Design review of the part built by this model. Coordinates are the model's own, in mm. Face numbers are marked on the shaded views. A direction names the side the tool comes from. Round coordinates to 2 decimals unless told otherwise and drop trailing zeros. Loops run counter-clockwise (first coordinate to the right, second up) from the corner with the lowest first, then second, coordinate; pieces in that order, holes last. Notation, with made-up numbers: (-5.75, -8.5) - (44.25, -8.5) arc R25 cw to (44.25, 26.5) - close; hole circle Ø11 at (35, 39.25). An arc over 180 degrees is marked (long way). Return JSON: item names as keys, results as strings. Group by question number.
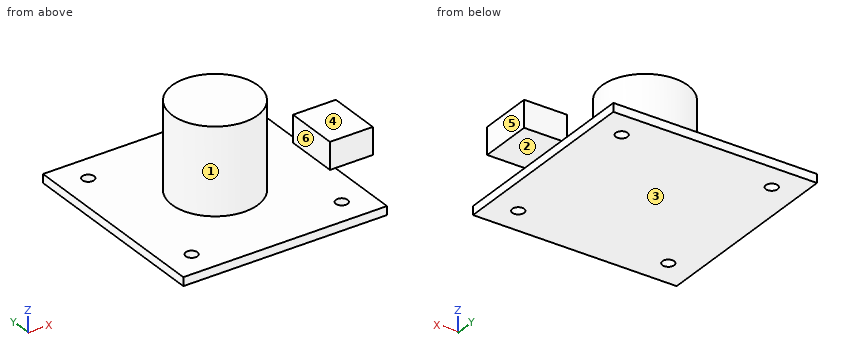
from build123d import *

# Parameters (mm, degrees)
SKETCH_1_W        = 38
SKETCH_1_H        = 38
SKETCH_1_R        = 1.1
USB_38_PCB_DEPTH  = 1.6
EXTRUDE_START     = 1.6
SKETCH_2_R        = 8
EXTRUDE_M12_DEPTH = 16
USB_START         = 1.6
SKETCH_3_W        = 8
SKETCH_3_H        = 10
USB_DEPTH         = 5


with BuildPart() as part:
    # 草图1 → USB摄像头38方PCB占位 (new body)
    with BuildSketch(Plane.XY):
        Rectangle(SKETCH_1_W, SKETCH_1_H)
        with Locations((-14, -14)):
            Circle(SKETCH_1_R, mode=Mode.SUBTRACT)
        with Locations((-14, 14)):
            Circle(SKETCH_1_R, mode=Mode.SUBTRACT)
        with Locations((14, -14)):
            Circle(SKETCH_1_R, mode=Mode.SUBTRACT)
        with Locations((14, 14)):
            Circle(SKETCH_1_R, mode=Mode.SUBTRACT)
    extrude(amount=USB_38_PCB_DEPTH)

    # 草图2 → M12镜头占位 (add)
    with BuildSketch(Plane.XY.offset(EXTRUDE_START)):
        Circle(SKETCH_2_R)
    extrude(amount=EXTRUDE_M12_DEPTH)

    # 草图3 → USB插头接口占位 (add)
    with BuildSketch(Plane.XY.offset(USB_START)):
        with Locations((22, 0)):
            Rectangle(SKETCH_3_W, SKETCH_3_H)
    extrude(amount=USB_DEPTH)


solid = part.part
Q1. Insertion check: pin 1 Ø0.5 at (y, z) = (2, 1) entering from +X; pin 2 Ø4 at (x, y) = (21.5, -1.5) entering from +Z; pin 3 Ø2.5 at (y, z) = (0, 5) entering from -X; pin 4 Ø7.5 at (x, y) = (21, 0) entering from -Z. Each pin has a flat end and moves straight along its axis. Give the tip position at first contact, or say it passes through.
Q2. Add section D-D, the plane y = 0. State the section outline as (x, z) points, plus the area to 3 significant figures.
Q3. Add section A-A, the plane y = 14. State the section outline as (x, z) points, plus the area to 3 significant figures.
Q4. Draft analysis for pull direction X (two halves, no side actions). For the marked faces 4, 5 and 6, state which applies: pulls with the +X half, pulls with the -X half, needs draft (parallel to the pull), parting line crosses it, or undercut.
Q5. Add section C-C, the plane z = 4.75. State the section outline as (x, y) points.
Q6. Tool access review of the marked faces 1, 2 and 3: name each direction out of +Z, -Z, +X, -X, +Y, -Y from which nothing blocks a thin tool from reaching the whole face with its end or side.
Q7. For line 1 (Y direction, x = -14, z = 0.95); line 2 (Z direction, x = 18, y = 13); line 3 (Z direction, x = 21, y = -2.5), list the stretches that pass through material, from the lowest coordinate up.
Evaluation:
{
 "1": {"pin 1": "x = 19", "pin 2": "z = 6.6", "pin 3": "x = -8", "pin 4": "z = 0"},
 "2": {"outline": "(-19, 0) - (19, 0) - (19, 1.6) - (26, 1.6) - (26, 6.6) - (18, 6.6) - (18, 1.6) - (8, 1.6) - (8, 17.6) - (-8, 17.6) - (-8, 1.6) - (-19, 1.6) - close", "area": "357 mm²"},
 "3": {"outline": "(-19, 0) - (-15.1, 0) - (-15.1, 1.6) - (-19, 1.6) - close; (-12.9, 0) - (12.9, 0) - (12.9, 1.6) - (-12.9, 1.6) - close; (15.1, 0) - (19, 0) - (19, 1.6) - (15.1, 1.6) - close", "area": "53.8 mm²"},
 "4": {"face 4": "needs draft", "face 5": "pulls with the +X half", "face 6": "undercut"},
 "5": {"outline": "circle Ø16 at (0, 0); (18, -5) - (26, -5) - (26, 5) - (18, 5) - close"},
 "6": {"face 1": "+Z", "face 2": "-Z, +X, +Y, -Y", "face 3": "-Z, +X, -X, +Y, -Y"},
 "7": {"line 1": "-19 to -15.1, -12.9 to 12.9, 15.1 to 19", "line 2": "0 to 1.6", "line 3": "1.6 to 6.6"}
}
